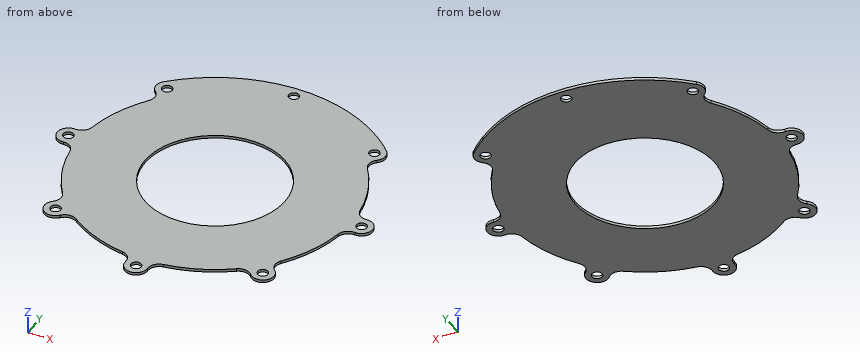
from build123d import *

# Parameters (mm, degrees)
NPTH_R              = 1.85
NPTH_R_2            = 25
BOSS_EXTRUDE1_DEPTH = 1


with BuildPart() as part:
    # NPTH → Boss-Extrude1 (new body)
    with BuildSketch(Plane.XY):
        with BuildLine():
            ThreePointArc((33.779497471, 45.912368166), (-4.301886792, 56.837432824), (-40.305086528, 40.305086528))
            ThreePointArc((-40.305086528, 40.305086528), (-41.47380633, 37.325608267), (-40.083553498, 34.442832912))
            ThreePointArc((-40.083553498, 34.442832912), (-38.716100837, 31.861298217), (-39.46852702, 29.03851537))
            ThreePointArc((-39.46852702, 29.03851537), (-45.270097093, 18.751488186), (-48.441794233, 7.375131965))
            ThreePointArc((-48.441794233, 7.375131965), (-49.90575747, 4.847077417), (-52.698113208, 3.988591777))
            ThreePointArc((-52.698113208, 3.988591777), (-57, 0), (-52.698113208, -3.988591777))
            ThreePointArc((-52.698113208, -3.988591777), (-49.90575747, -4.847077417), (-48.441794233, -7.375131965))
            ThreePointArc((-48.441794233, -7.375131965), (-45.270097093, -18.751488186), (-39.46852702, -29.03851537))
            ThreePointArc((-39.46852702, -29.03851537), (-38.716100837, -31.861298217), (-40.083553498, -34.442832912))
            ThreePointArc((-40.083553498, -34.442832912), (-40.305086528, -40.305086528), (-34.442832912, -40.083553498))
            ThreePointArc((-34.442832912, -40.083553498), (-31.861298217, -38.716100837), (-29.03851537, -39.46852702))
            ThreePointArc((-29.03851537, -39.46852702), (-18.751488186, -45.270097093), (-7.375131965, -48.441794233))
            ThreePointArc((-7.375131965, -48.441794233), (-4.847077417, -49.90575747), (-3.988591777, -52.698113208))
            ThreePointArc((-3.988591777, -52.698113208), (0, -57), (3.988591777, -52.698113208))
            ThreePointArc((3.988591777, -52.698113208), (4.847077417, -49.90575747), (7.375131965, -48.441794233))
            ThreePointArc((7.375131965, -48.441794233), (18.751488186, -45.270097093), (29.03851537, -39.46852702))
            ThreePointArc((29.03851537, -39.46852702), (31.861298217, -38.716100837), (34.442832912, -40.083553498))
            ThreePointArc((34.442832912, -40.083553498), (40.305086528, -40.305086528), (40.083553498, -34.442832912))
            ThreePointArc((40.083553498, -34.442832912), (38.716100837, -31.861298217), (39.46852702, -29.03851537))
            ThreePointArc((39.46852702, -29.03851537), (45.270097093, -18.751488186), (48.441794233, -7.375131965))
            ThreePointArc((48.441794233, -7.375131965), (49.90575747, -4.847077417), (52.698113208, -3.988591777))
            ThreePointArc((52.698113208, -3.988591777), (57, 0), (52.698113208, 3.988591777))
            ThreePointArc((52.698113208, 3.988591777), (49.90575747, 4.847077417), (48.441794233, 7.375131965))
            ThreePointArc((48.441794233, 7.375131965), (45.270097093, 18.751488186), (39.46852702, 29.03851537))
            ThreePointArc((39.46852702, 29.03851537), (38.716100837, 31.861298217), (40.083553498, 34.442832912))
            ThreePointArc((40.083553498, 34.442832912), (41.47380633, 37.325608267), (40.305086528, 40.305086528))
            ThreePointArc((40.305086528, 40.305086528), (37.148240852, 43.232027498), (33.779497471, 45.912368166))
        make_face()
        with Locations((-37.476659403, -37.476659403)):
            Circle(NPTH_R, mode=Mode.SUBTRACT)
        with Locations((-53, 0)):
            Circle(NPTH_R, mode=Mode.SUBTRACT)
        with Locations((0, -53)):
            Circle(NPTH_R, mode=Mode.SUBTRACT)
        with Locations((37.476659403, -37.476659403)):
            Circle(NPTH_R, mode=Mode.SUBTRACT)
        Circle(NPTH_R_2, mode=Mode.SUBTRACT)
        with Locations((53, 0)):
            Circle(NPTH_R, mode=Mode.SUBTRACT)
        with Locations((-37.476659403, 37.476659403)):
            Circle(NPTH_R, mode=Mode.SUBTRACT)
        with Locations((0, 53)):
            Circle(NPTH_R, mode=Mode.SUBTRACT)
        with Locations((37.476659403, 37.476659403)):
            Circle(NPTH_R, mode=Mode.SUBTRACT)
    extrude(amount=BOSS_EXTRUDE1_DEPTH)


solid = part.part
The listing builds one solid part. Answer for the finished solid, in the listing's coordinates (mm). Give positions to 0.01 mm unless a question says otherwise; leave off trailing zeros. Loops run counter-clockwise (first coordinate to the right, second up) from the corner with the lowest first, then second, coordinate; pieces in that order, holes last. Notation, with made-up numbers: (19, -21) - (43, -21) arc R27 ccw to (43, 5) - close; hole circle Ø7 at (17, -26). An arc over 180 degrees is marked (long way). Answer as a JSON object with one key per item and string values.
1. A flat-ended cylindrical pin translates along its axis: pin 1 Ø5 at (x, y) = (-37.48, 37.48) entering from +Z. Find the tip coordinate at first contact, or state that the pin passes through.
Determined:
{"pin 1": "z = 1"}
2. Find the intervals of material crossed by L1, parallel to Y at x = 0, z = 0.7; L2, parallel to Y at x = 53, z = 0.55; L3, parallel to X at y = 38, z = 0.7, in increasing order. Write a range as [from, to].
Determined:
{"L1": "[-57, -54.85], [-51.15, -25], [25, 51.15], [54.85, 57]", "L2": "[-4, -1.85], [1.85, 4]", "L3": "[-41.44, -39.25], [-35.7, 35.7], [39.25, 41.44]"}
3. A cutting plane is placed at D-D (z = 0.7). Give the number of separate pieces and of enclosed holes in the cut face, then the cut area to 3 significant figures.
Determined:
{"separate pieces": "1", "enclosed holes": "9", "area": "6,530 mm²"}
4. A cutting plane is placed at A-A (x = 0). Write down the section's boundary in (y, z), then the cut area to 3 significant figures.
Determined:
{"outline": "(-57, 0) - (-54.85, 0) - (-54.85, 1) - (-57, 1) - close; (-51.15, 0) - (-25, 0) - (-25, 1) - (-51.15, 1) - close; (25, 0) - (51.15, 0) - (51.15, 1) - (25, 1) - close; (54.85, 0) - (57, 0) - (57, 1) - (54.85, 1) - close", "area": "56.6 mm²"}
5. A cutting plane is placed at C-C (y = -20). Write down the section's boundary in (x, z).
Determined:
{"outline": "(-44.73, 0) - (-15, 0) - (-15, 1) - (-44.73, 1) - close; (15, 0) - (44.73, 0) - (44.73, 1) - (15, 1) - close"}
